Can you work these out from the model? Positions are in its coordinate system, mm. A direction names the side the tool comes from. Coordinates: 2 decimals unless noted, no trailing zeros. Loops run counter-clockwise (first coordinate to the right, second up) from the corner with the lowest first, then second, coordinate; pieces in that order, holes last. Notation, with made-up numbers: (88, -39) -> (135, -39) arc R22 cw to (135, -15) -> close; hole circle Ø10 at (69.5, -11). An arc over 180 degrees is marked (long way). Put each result on its own line as item: value. Start each with the question number.
Item 1: If we section it at B-B on x = -70.5: Please give me the cut outline in (y, z), plus the area to 4 significant figures.
Item 2: We'd pull the mould along X, two halves only. Please class faces 1 (the flat face through (-65, 10, 87)), 2 (the cylindrical face through (-14.86, 17.6, 4.06)), 3 (the cylindrical face through (-75.14, 17.6, 3.94)): pulls with the +X half, pulls with the -X half, needs draft (parallel to the pull), parting line crosses it, or undercut.
Item 3: Will these pins go through, and if not, where does the flat tip stop? P1, Ø2, axis at x = -60.5, z = 51, coming from the +Y side; P2, Ø1.5, axis at x = -44.5, y = 2.5, coming from the -Z side.
Item 4: For faces 4 (the flat face through (-72, 12, 83.5)), 5 (the cylindrical face through (-65.86, 17.6, 4.06)), 6 (the cylindrical face through (-50.573, 2.465, 23.412)), which set-ups out of +Z, -Z, +X, -X, +Y, -Y let a thin tool reach every point of the face, with its end or its side?
Item 5: If we section it at C-C on y = 13: State how many separate pieces and enclosed holes the cut face has, plus the area to 3 significant figures.
Item 6: Please list where these lines run through material, in increasing order: L1, parallel to X at y = 3.3, z = 67.75 (3 decimals); L2, parallel to Z at x = -49.5, y = 1.2 (3 decimals); L3, parallel to Z at x = -17.5, y = 6. Write a range as from..to.
Item 7: If we section it at A-A on z = 23.75: Please give me the cut outline in (x, y) (3 decimals).
Item 8: If we section it at D-D on y = 8.75: Please give me the cut outline in (x, z), plus the area to 3 significant figures.
Autodesk Inventor part; units mm, degrees
ref_plane "YZ Plane" through (0, 0, 0) normal (1, 0, 0) x (0, 1, 0)
ref_plane "XZ Plane" through (0, 0, 0) normal (0, 1, 0) x (-1, 0, 0)
ref_plane "XY Plane" through (0, 0, 0) normal (0, 0, 1) x (1, 0, 0)
sketch "Sketch1" plane through (0, 0, 0) normal (0, 1, 0) x (-1, 0, 0)
  line L0 (14, 91.5) -> (76, 91.5)
  line L1 (45, 91.5) -> (45, 1.5) construction
  circle A0 centre (49.5, 67.75) radius 1.125
  circle A1 centre (49.5, 23.75) radius 1.125
  line L2 (0, 45.75) -> (90, 45.75) construction
  circle A2 centre (40.5, 67.75) radius 1.125
  circle A3 centre (40.5, 23.75) radius 1.125
  line L3 (37.5, 20) -> (37.5, 0)
  line L4 (52.5, 20) -> (52.5, 0)
  line L5 (76, 0) -> (52.5, 0)
  line L6 (37.5, 0) -> (0, 0)
  line L7 (52.5, 20) -> (37.5, 20)
  line L8 (14, 0) -> (14, 91.5)
  line L9 (76, 0) -> (76, 91.5)
  dimension "d4" = 2.25
  dimension "d5" = 2.25
  dimension "d6" = 22
  dimension "d7" = 22
  dimension "d8" = 4.5
  dimension "d9" = 4.5
  dimension "d45" = 20
extrude "Extrusion1" add sketch "Sketch1" along normal blind 5
sketch "Sketch4" plane through (0, 5, 0) normal (0, 1, 0) x (1, 0, 0)
  line L0 (-37.5, -20) -> (-52.5, -20)
  line L1 (-76, -91.5) -> (-14, -91.5)
  line L2 (-45, -91.5) -> (-45, -20) construction
  line L3 (-25, -83.5) -> (-14, -83.5)
  line L4 (-14, -83.5) -> (-14, -91.5)
  line L5 (-14, -91.5) -> (-25, -91.5)
  line L6 (-25, -91.5) -> (-25, -83.5)
  dimension "d28" = 11
  dimension "d29" = 8
  dimension "d30" = 0
  dimension "d31" = 20
extrude "Extrusion4" add sketch "Sketch4" along normal blind 13.5
sketch "Sketch5" plane through (-14, 5, 83.5) normal (0, 0, -1) x (-1, 0, 0)
  line L0 (11, 0) -> (11, 13.5)
  line L1 (0, 13.5) -> (11, 13.5)
  circle A0 centre (5.5, 8) radius 1.5
  point P0 (-14, -5)
  dimension "d34" = 3
  dimension "d35" = 5.5
  dimension "d36" = 5.5
extrude "Extrusion5" cut sketch "Sketch5" against normal blind 8
fillet "Fillet1" radius 3 2 edges at (-14, 18.5, 87.5) (-25, 18.5, 87.5)
pattern_linear "Rectangular Pattern4" count 2 spacing 83.5 along (0, 0, -1) count 2 spacing 51 along (-1, 0, 0) of "Extrusion4", "Fillet1", "Extrusion5"
properties part number "Base1"
Solutions:
1. outline: (0, 0) -> (11.5, 0) -> (11.5, 8) -> (5, 8) -> (5, 83.5) -> (11.5, 83.5) -> (11.5, 91.5) -> (0, 91.5) -> close; (14.5, 0) -> (18.5, 0) -> (18.5, 8) -> (14.5, 8) -> close; (14.5, 83.5) -> (18.5, 83.5) -> (18.5, 91.5) -> (14.5, 91.5) -> close
1. area: 625.5 mm^2
2. face 1: undercut
2. face 2: pulls with the +X half
2. face 3: pulls with the -X half
3. P1: y = 5
3. P2: z = 20
4. face 4: +X, -X, +Y
4. face 5: +Z, -Z, +Y
4. face 6: +Y, -Y
5. separate pieces: 8
5. enclosed holes: 0
5. area: 256 mm^2
6. L1: -76..-50.625, -48.375..-41.625, -39.375..-14
6. L2: 20..22.625, 24.875..66.625, 68.875..91.5
6. L3: 0..8, 83.5..91.5
7. outline: (-76, 0) -> (-50.625, 0) -> (-50.625, 5) -> (-76, 5) -> close; (-48.375, 0) -> (-41.625, 0) -> (-41.625, 5) -> (-48.375, 5) -> close; (-39.375, 0) -> (-14, 0) -> (-14, 5) -> (-39.375, 5) -> close
8. outline: (-76, 0) -> (-65, 0) -> (-65, 8) -> (-76, 8) -> close; (-76, 83.5) -> (-65, 83.5) -> (-65, 91.5) -> (-76, 91.5) -> close; (-25, 0) -> (-14, 0) -> (-14, 8) -> (-25, 8) -> close; (-25, 83.5) -> (-14, 83.5) -> (-14, 91.5) -> (-25, 91.5) -> close
8. area: 352 mm^2
